Here's the drawing with two shaded views (mm, measured from the low corner). I have some questions. A direction names the side the tool comes from. Coordinates: 2 decimals unless noted, no trailing zeros. Loops run counter-clockwise (first coordinate to the right, second up) from the corner with the lowest first, then second, coordinate; pieces in that order, holes last. Notation, with made-up numbers: (22, 78.5) - (77, 78.5) arc R14 ccw to (77, 105.5) - close; hole circle Ø2 at (14, -1.75). An arc over 180 degrees is marked (long way). One line per item, written item: value. Start each with the question number.
(1) I'm going to push flat-ended pins straight in: P1, Ø0.9, axis at y = 4.5, z = 2, coming from the +X side; P2, Ø1, axis at x = 19, z = 2.5, coming from the +Y side; P3, Ø1.5, axis at x = 24.5, z = 2, coming from the -Y side. Where does each tip first touch, or does it pass through?
(2) If we mould it in two halves opening along Y, with no side actions, what happens to the marked faces 6, 7, 8 and 9? For each: pulls with the +Y half, pulls with the -Y half, needs draft (parallel to the pull), parting line crosses it, or undercut.
(3) If we section it at D-D on y = 21.5: Write out the boundary of the cut face in (x, z), then the cut area to 3 significant figures.
(4) If we section it at A-A on y = 7: Write out the boundary of the cut face in (x, z), then the cut area to 3 significant figures.
(5) If we section it at B-B on z = 2.3: Write out the boundary of the cut face in (x, y).
(6) If we section it at C-C on x = 14.1: Write out the boundary of the cut face in (y, z).
(7) If I drill on line 1 along Y through (x, z) = (14.1, 0.6); line 2 along X through (y, z) = (23.25, 0.6); line 3 along X through (y, z) = (25, 1.45), over which ranges is the centre line in solid material (lowest first)? Write a range as from..to.
(8) On a 3-axis mill with a long thin cutter (end or side, diameter ignored), from which of +Z, -Z, +X, -X, +Y, -Y can I reach the whole of each face in a straight line? I mean the marked faces 1, 2, 3, 4 and 5. Say none if no direction works.
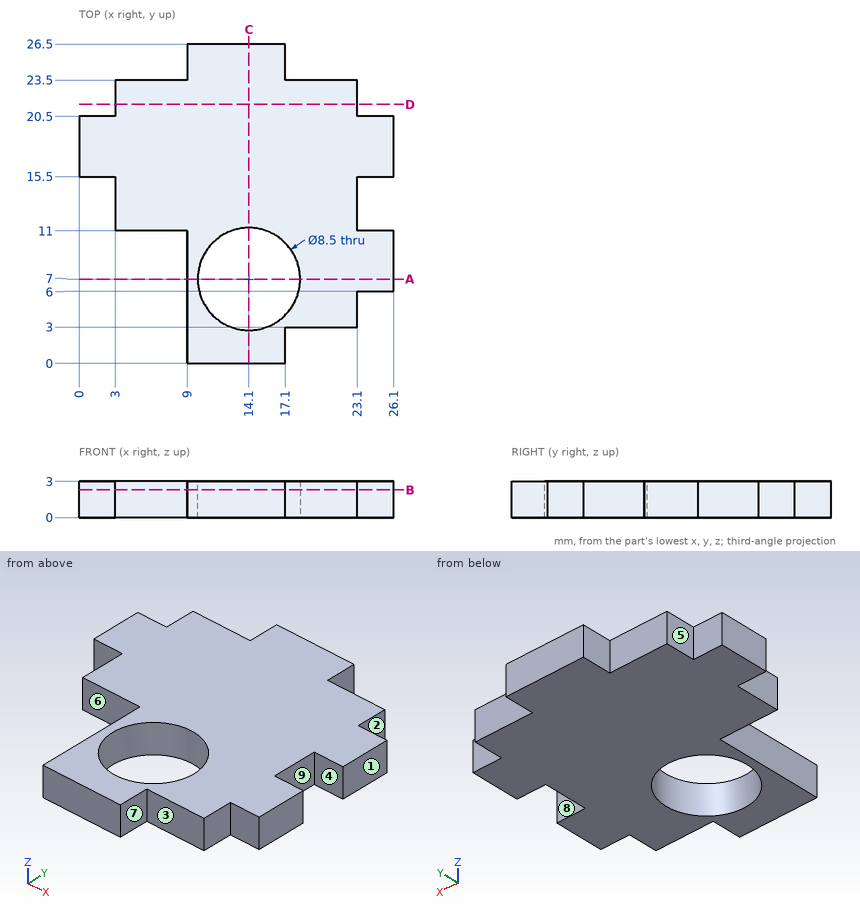
Values:
1. P1: stops at x = 23.1
1. P2: stops at y = 23.5
1. P3: stops at y = 6
2. face 6: pulls with the -Y half
2. face 7: needs draft
2. face 8: undercut
2. face 9: undercut
3. outline: (3, 0) - (23.1, 0) - (23.1, 3) - (3, 3) - close
3. area: 60.3 mm2
4. outline: (9, 0) - (9.85, 0) - (9.85, 3) - (9, 3) - close; (18.35, 0) - (26.1, 0) - (26.1, 3) - (18.35, 3) - close
4. area: 25.8 mm2
5. outline: (0, 15.5) - (3, 15.5) - (3, 11) - (9, 11) - (9, 0) - (17.1, 0) - (17.1, 3) - (23.1, 3) - (23.1, 6) - (26.1, 6) - (26.1, 11) - (23.1, 11) - (23.1, 15.5) - (26.1, 15.5) - (26.1, 20.5) - (23.1, 20.5) - (23.1, 23.5) - (17.1, 23.5) - (17.1, 26.5) - (9, 26.5) - (9, 23.5) - (3, 23.5) - (3, 20.5) - (0, 20.5) - close; hole circle Ø8.5 at (14.1, 7)
6. outline: (0, 0) - (2.75, 0) - (2.75, 3) - (0, 3) - close; (11.25, 0) - (26.5, 0) - (26.5, 3) - (11.25, 3) - close
7. line 1: y = 0..2.75, 11.25..26.5
7. line 2: x = 3..23.1
7. line 3: x = 9..17.1
8. face 1: +Z, -Z, +X, +Y, -Y
8. face 2: +Z, -Z, +X, +Y
8. face 3: +Z, -Z, +X, -Y
8. face 4: +Z, -Z, +X
8. face 5: +Z, -Z, -X, +Y
